Autodesk Inventor part; units mm, degrees
ref_plane "Plano de trabalho1" through (0, 12.85, 9.2) normal (0, 0, 1) x (1, 0, 0)
ref_plane "Plano de trabalho2" through (-9.2, 12.85, 0) normal (1, 0, 0) x (0, 1, 0)
ref_plane "XZ Plane" through (0, 0, 0) normal (0, 1, 0) x (-1, 0, 0)
sketch "Esboço1" plane through (0, 0, 0) normal (0, 0, 1) x (1, 0, 0)
  line L0 (0, 0) -> (7.3, 0)
  line L1 (7.3, 0) -> (7.3, 2.85)
  line L2 (7.3, 2.85) -> (9.2, 2.85)
  line L3 (0, 22.85) -> (0, 0)
  line L4 (9.2, 2.85) -> (9.2, 6.85)
  line L5 (6.85, 0) -> (6.85, 22.85)
  line L6 (9.2, 6.85) -> (9.2, 22.85)
  line L7 (9.2, 6.85) -> (9.2, 6.85)
  line L8 (9.2, 22.85) -> (0, 22.85)
  dimension "d0" = 7.3
  dimension "d1" = 2.85
  dimension "d4" = 4
  dimension "d7" = 9.2
  dimension "d11" = 2.35
  dimension "d12" = 9.2
  dimension "d24" = 16
revolve "Revolução1" add sketch "Esboço1" angle 360 about axis through (0, 22.85, 0) along (0, -1, 0) contours L5 L8 L6 L4 L2 L1 L0
ref_plane "Plano de trabalho1" through (0, 12.85, 9.2) normal (0, 0, 1) x (1, 0, 0)
sketch "Esboço3" plane through (0, 12.85, 9.2) normal (0, 0, 1) x (1, 0, 0)
  line L0 (0, -12.85) -> (0, -6.85)
  line L1 (-9.2, 10) -> (9.2, 10)
  line L2 (0, -6.85) -> (0, -4.35)
  arc A0 (-2.5, -4.35) -> (2.5, -4.35) centre (0, -4.35) ccw
  line L3 (2.5, -4.35) -> (2.5, 10)
  line L4 (-2.5, -4.35) -> (-2.5, 10)
  point P0 (-2, 10)
  point P1 (2, 10)
  dimension "d16" = 6
  dimension "d25" = 2.5
ref_plane "Plano de trabalho2" through (-9.2, 12.85, 0) normal (1, 0, 0) x (0, 1, 0)
sketch "Esboço4" plane through (-9.2, 12.85, 0) normal (1, 0, 0) x (0, 1, 0)
  line L0 (-12.85, 0) -> (-6.85, 0)
  line L1 (10, 0) -> (10, 0)
  line L2 (10, -2) -> (10, 2)
  line L3 (10, 0) -> (10, 0)
  arc A0 (-4.35, 2.5) -> (-4.35, -2.5) centre (-4.35, 0) ccw
  line L4 (-4.35, 2.5) -> (10, 2.5)
  line L5 (-4.35, -2.5) -> (10, -2.5)
  line L6 (10, -2.5) -> (10, 2.5)
  dimension "d20" = 6
extrude "Extrusão3" cut sketch "Esboço3" against normal blind 20
extrude "Extrusão4" cut sketch "Esboço4" along normal blind 20
properties part number "trava_botao_3DPrint"
Verification items for the finished model (mm, model axes). A direction names the side the tool comes from. Coordinates: 2 decimals unless noted, no trailing zeros. Write each loop counter-clockwise with the first axis right and the second up, starting at its lowest first coordinate (ties: lowest second). Pieces come first, ordered by that corner, then holes. Notation, with made-up numbers: M 84,-18 L 99,-18 A11 ccw 99,-9 Z; hole C -20.75,10 d7. An arc over 180 degrees is marked long. One line per question, with ' | ' between items.
1) Depth check by flat-ended pin: pin 1 Ø2 at (x, y) = (-8, 14.5) entering from -Z; pin 2 Ø0.7 at (y, z) = (14.5, -7.5) entering from -X; pin 3 Ø1.5 at (y, z) = (19, 7) entering from -X. Enter the tip coordinate at first touch or a pass-through.
Solutions:
pin 1: z = -5.97 | pin 2: x = -5.79 | pin 3: x = -6.75
2) Sectioned sample at C-C on y = 15. Record the cut outline in (x, z), then the cut area to 3 significant figures.
Solutions:
outline: M -8.85,-2.5 A9.2 ccw -2.5,-8.85 L -2.5,-6.38 A6.85 cw -6.38,-2.5 Z; M -8.85,2.5 L -6.38,2.5 A6.85 cw -2.5,6.38 L -2.5,8.85 A9.2 ccw Z; M 2.5,-8.85 A9.2 ccw 8.85,-2.5 L 6.38,-2.5 A6.85 cw 2.5,-6.38 Z; M 2.5,6.38 A6.85 cw 6.38,2.5 L 8.85,2.5 A9.2 ccw 2.5,8.85 Z | area: 70.7 mm^2
3) Access from +Z, -Z, +X, -X, +Y, -Y to the whole of each face (thin tool, end or side, straight path). Record for faces 1 (the face through (3.161, 9.046, 6.077)), 2 (the face through (8, 16, 2.5)), 3 (the face through (-3, 2.85, 7)), 4 (the face through (2.5, 16, -8)).
Solutions:
face 1: +Y, -Y | face 2: +X, -X, +Y | face 3: -Y | face 4: +Z, -Z, +Y
4) Release check for a two-part mould opening along X. For faces 5 (the face through (6.963, 1.445, -2.193)), 6 (the face through (-8, 16, 2.5)), 7 (the face through (-2.5, 16, -8)) record: +X half, -X half, draft (parallel to the pull), parting line (faces both ways), or undercut.
Solutions:
face 5: parting line | face 6: draft | face 7: undercut
5) Sectioned sample at A-A on z = 0. Record the cut outline in (x, y).
Solutions:
outline: M -9.2,2.85 L -7.3,2.85 L -7.3,0 L -6.85,0 L -6.85,6 L -9.2,6 Z; M 6.85,0 L 7.3,0 L 7.3,2.85 L 9.2,2.85 L 9.2,6 L 6.85,6 Z
6) Material ranges on L1, parallel to Z at x = 0, y = 5.5; L2, parallel to Y at x = -6.25, z = -5.75; L3, parallel to Z at x = 4.75, y = 4.25, recorded low to high.
Solutions:
L1: -9.2 to -6.85, 6.85 to 9.2 | L2: 2.85 to 22.85 | L3: -7.88 to -4.94, 4.94 to 7.88
7) Sectioned sample at B-B on x = 0. Record the cut outline in (y, z), then the cut area to 3 significant figures.
Solutions:
outline: M 0,-7.3 L 2.85,-7.3 L 2.85,-9.2 L 6,-9.2 L 6,-6.85 L 0,-6.85 Z; M 0,6.85 L 6,6.85 L 6,9.2 L 2.85,9.2 L 2.85,7.3 L 0,7.3 Z | area: 17.4 mm^2
